Design review of the part built by this model. Coordinates are the model's own, in mm. A direction names the side the tool comes from. Coordinates: 2 decimals unless noted, no trailing zeros. Write each loop counter-clockwise with the first axis right and the second up, starting at its lowest first coordinate (ties: lowest second). Pieces come first, ordered by that corner, then holes. Notation, with made-up numbers: (59.5, 44.5) -> (103.5, 44.5) arc R32 ccw to (103.5, 73.5) -> close; hole circle Ø2 at (55, -36.75). An arc over 180 degrees is marked (long way). Write item = value, one per line. Start each with the question number.
```python
from build123d import *

# Parameters (mm, degrees)
SKETCH2_W                       = 63.5
SKETCH2_H                       = 63.5
BOSS_EXTRUDE2_DEPTH             = 6.35
SKETCH3_W                       = 25.4
SKETCH3_H                       = 25.4
BOSS_EXTRUDE3_DEPTH             = 76.2
SKETCH14_W                      = 59.944
SKETCH14_H                      = 59.944
BOSS_EXTRUDE6_DEPTH             = 6.35
CBORE_FOR_M6_SBHCS2_D           = 6.6
CBORE_FOR_M6_SBHCS2_DEPTH       = 7.62
CBORE_FOR_M6_SBHCS2_CBORE_D     = 10
CBORE_FOR_M6_SBHCS2_CBORE_DEPTH = 3.3
CBORE_FOR_M6_SBHCS2_TIP         = 1.982840043
TAP_DRILL_FOR_M3X0_5_TAP2_D     = 2.5
TAP_DRILL_FOR_M3X0_5_TAP2_DEPTH = 7.62
TAP_DRILL_FOR_M3X0_5_TAP2_TIP   = 0.751075774


with BuildPart() as part:
    # Sketch2 → Boss-Extrude2 (new body)
    with BuildSketch(Plane.XY):
        with Locations((31.75, 31.75)):
            Rectangle(SKETCH2_W, SKETCH2_H)
    extrude(amount=BOSS_EXTRUDE2_DEPTH)

    # Sketch3 → Boss-Extrude3 (add)
    with BuildSketch(Plane.XY.offset(6.35)):
        with Locations((31.75, 31.75)):
            Rectangle(SKETCH3_W, SKETCH3_H)
    extrude(amount=BOSS_EXTRUDE3_DEPTH)

    # Sketch14 → Boss-Extrude6 (add)
    with BuildSketch(Plane.XY.offset(82.55)):
        with Locations((31.75, 31.75)):
            Rectangle(SKETCH14_W, SKETCH14_H)
    extrude(amount=BOSS_EXTRUDE6_DEPTH)

    # CBORE for M6 SBHCS2
    with Locations(Plane.XY.offset(6.35)):
        with Locations((57.15, 31.75), (31.75, 6.35), (31.75, 57.15), (6.35, 31.75)):
            CounterBoreHole(CBORE_FOR_M6_SBHCS2_D / 2, CBORE_FOR_M6_SBHCS2_CBORE_D / 2, CBORE_FOR_M6_SBHCS2_CBORE_DEPTH, depth=CBORE_FOR_M6_SBHCS2_DEPTH)
            with Locations((0, 0, -(CBORE_FOR_M6_SBHCS2_DEPTH + CBORE_FOR_M6_SBHCS2_TIP / 2))):  # 118° drill point
                Cone(0, CBORE_FOR_M6_SBHCS2_D / 2, CBORE_FOR_M6_SBHCS2_TIP, mode=Mode.SUBTRACT)

    # Tap Drill for M3x0.5 Tap2
    with Locations(Plane.XY.offset(88.9)):
        with Locations((9.271, 51.816), (9.271, 11.684), (54.229, 11.684), (54.229, 51.816), (11.684, 39.243), (11.684, 24.257), (51.816, 39.243), (51.816, 24.257)):
            Hole(TAP_DRILL_FOR_M3X0_5_TAP2_D / 2, depth=TAP_DRILL_FOR_M3X0_5_TAP2_DEPTH)
            with Locations((0, 0, -(TAP_DRILL_FOR_M3X0_5_TAP2_DEPTH + TAP_DRILL_FOR_M3X0_5_TAP2_TIP / 2))):  # 118° drill point
                Cone(0, TAP_DRILL_FOR_M3X0_5_TAP2_D / 2, TAP_DRILL_FOR_M3X0_5_TAP2_TIP, mode=Mode.SUBTRACT)


solid = part.part
```
(1) Take a section at D-D, the plane z = 35.5. State the section outline as (x, y) points.
(2) For line 1 (Y direction, x = 31.75, z = 1.4); line 2 (Z direction, x = 55.5, y = 22); line 3 (Z direction, x = 57.5, y = 27), list the stretches that pass through material, from the lowest coordinate up.
(3) Take a section at B-B, the plane x = 57.15. State the section outline as (y, z) points, then the cut area to 3 significant figures.
(4) Take a section at A-A, the plane y = 48. State the section outline as (x, z) points.
(5) Mouldability with a two-part tool opening along Y and no side actions: class faces 1 (the face through (51.14, 25.31, 85.68)), 2 (the face through (44.45, 32, 44)), 3 (the face through (31, 61.722, 86)) as pulls with the +Y half, pulls with the -Y half, needs draft (parallel to the pull), parting line crosses it, or undercut.
(6) For pin 1 Ø2 at (x, y) = (9.271, 51.816) entering from +Z; pin 2 Ø3 at (y, z) = (39, 66) entering from +X; pin 3 Ø10 at (x, z) = (24.5, 66.5) entering from +Y, all flat-tipped, find the tip position at first contact; note any pin that passes through.
(7) For faces 4 (the face through (1.778, 31, 86)), 5 (the face through (11.01, 25.31, 85.68)), 6 (the face through (26.755, 6.57, 4.723)), list the 3-axis set-ups (+Z, -Z, +X, -X, +Y, -Y) from which the entire face can be reached by the end or side of a thin tool; tool diameter is ignored.
Report:
q1.outline = (19.05, 19.05) -> (44.45, 19.05) -> (44.45, 44.45) -> (19.05, 44.45) -> close
q2.line_1 = 0 to 3.05, 9.65 to 53.85, 60.45 to 63.5
q2.line_2 = 0 to 6.35, 82.55 to 88.9
q2.line_3 = 0 to 3.05, 82.55 to 88.9
q3.outline = (0, 0) -> (28.45, 0) -> (28.45, 3.05) -> (26.75, 3.05) -> (26.75, 6.35) -> (0, 6.35) -> close; (1.78, 82.55) -> (61.72, 82.55) -> (61.72, 88.9) -> (1.78, 88.9) -> close; (35.05, 0) -> (63.5, 0) -> (63.5, 6.35) -> (36.75, 6.35) -> (36.75, 3.05) -> (35.05, 3.05) -> close
q3.area = 731 mm2
q4.outline = (0, 0) -> (63.5, 0) -> (63.5, 6.35) -> (0, 6.35) -> close; (1.78, 82.55) -> (61.72, 82.55) -> (61.72, 88.9) -> (1.78, 88.9) -> close
q5.face_1 = undercut
q5.face_2 = needs draft
q5.face_3 = pulls with the +Y half
q6.pin_1 = 6.35
q6.pin_2 = 44.45
q6.pin_3 = 44.45
q7.face_4 = +Z, -X, +Y, -Y
q7.face_5 = +Z
q7.face_6 = none
